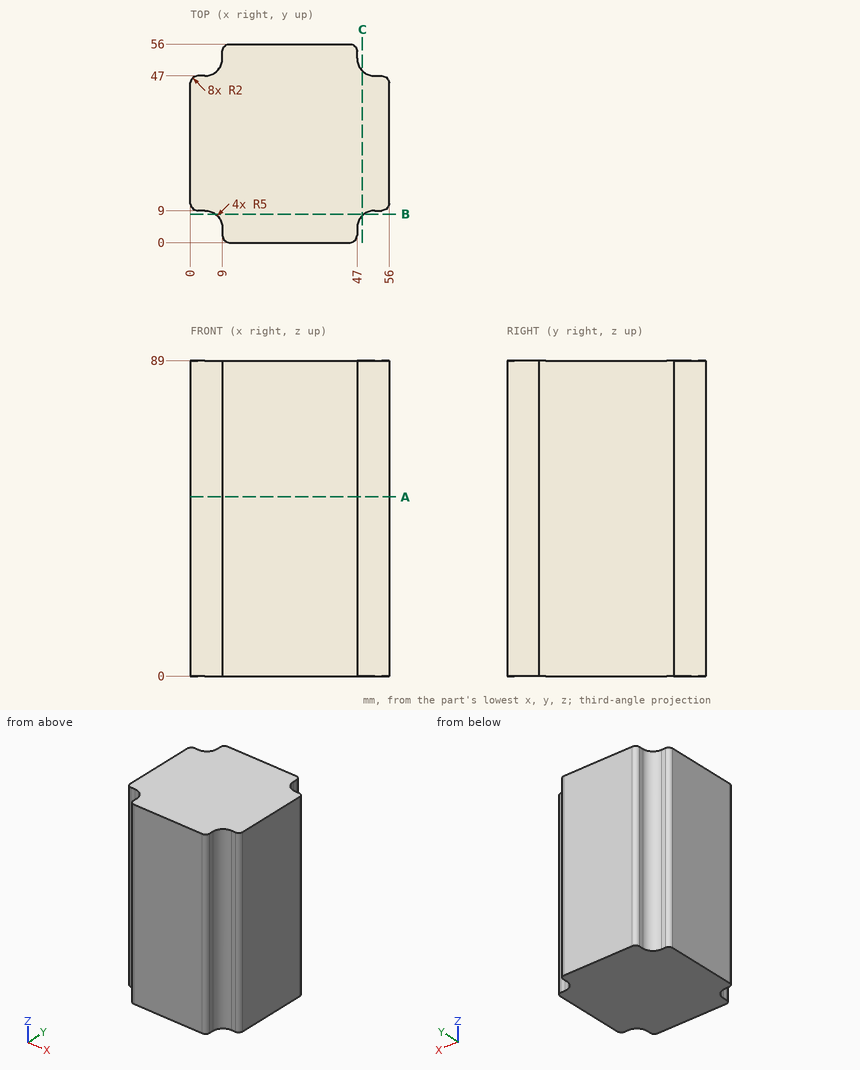
Geometry: see drawing. Coordinates: mm, zero at the bounding-box minimum. Round coordinates to 2 decimals unless told otherwise and drop trailing zeros. Write each loop counter-clockwise with the first axis right and the second up, starting at its lowest first coordinate (ties: lowest second). Pieces come first, ordered by that corner, then holes.
1) Contact query for flat-ended pins moving along their axis: P1, Ø2, axis at x = 53, z = 50.5, coming from the -Y side; P2, Ø2, axis at x = 49, z = 67, coming from the -Y side; P3, Ø1.6, axis at x = 3, z = 24, coming from the +Y side. Output: stop coordinate, or through.
2) Ray query, L1, parallel to Y at x = 52.5, z = 11; L2, parallel to Y at x = 51, z = 6.5; L3, parallel to X at y = 6.5, z = 66. Return the intervals inside material, ascending.
3) Cut plane C-C (x = 48.5). Return the cut outline in (y, z), then the cut area to 3 significant figures.
4) Cut plane B-B (y = 8). Return the cut outline in (x, z), then the cut area to 3 significant figures.
5) Cut plane A-A (z = 50.5). Return the cut outline in (x, y), then the cut area to 3 significant figures.
Geometry says:
1. P1: stops at y = 9
1. P2: stops at y = 7
1. P3: stops at y = 47
2. L1: y = 9 to 47
2. L2: y = 8.9 to 47.1
2. L3: x = 8.33 to 47.67
3. outline: (7.57, 0) - (48.43, 0) - (48.43, 89) - (7.57, 89) - close
3. area: 3,640 mm2
4. outline: (7, 0) - (49, 0) - (49, 89) - (7, 89) - close
4. area: 3,740 mm2
5. outline: (0, 11) arc R2 ccw to (2, 9) - (4, 9) arc R5 cw to (9, 4) - (9, 2) arc R2 ccw to (11, 0) - (45, 0) arc R2 ccw to (47, 2) - (47, 4) arc R5 cw to (52, 9) - (54, 9) arc R2 ccw to (56, 11) - (56, 45) arc R2 ccw to (54, 47) - (52, 47) arc R5 cw to (47, 52) - (47, 54) arc R2 ccw to (45, 56) - (11, 56) arc R2 ccw to (9, 54) - (9, 52) arc R5 cw to (4, 47) - (2, 47) arc R2 ccw to (0, 45) - close
5. area: 2,830 mm2
